For this review, use the dimensioned drawing (mm, ordinates from the lowest corner) and the shaded views. A direction names the side the tool comes from. Coordinates: 2 decimals unless noted, no trailing zeros. Write each loop counter-clockwise with the first axis right and the second up, starting at its lowest first coordinate (ties: lowest second). Pieces come first, ordered by that corner, then holes.
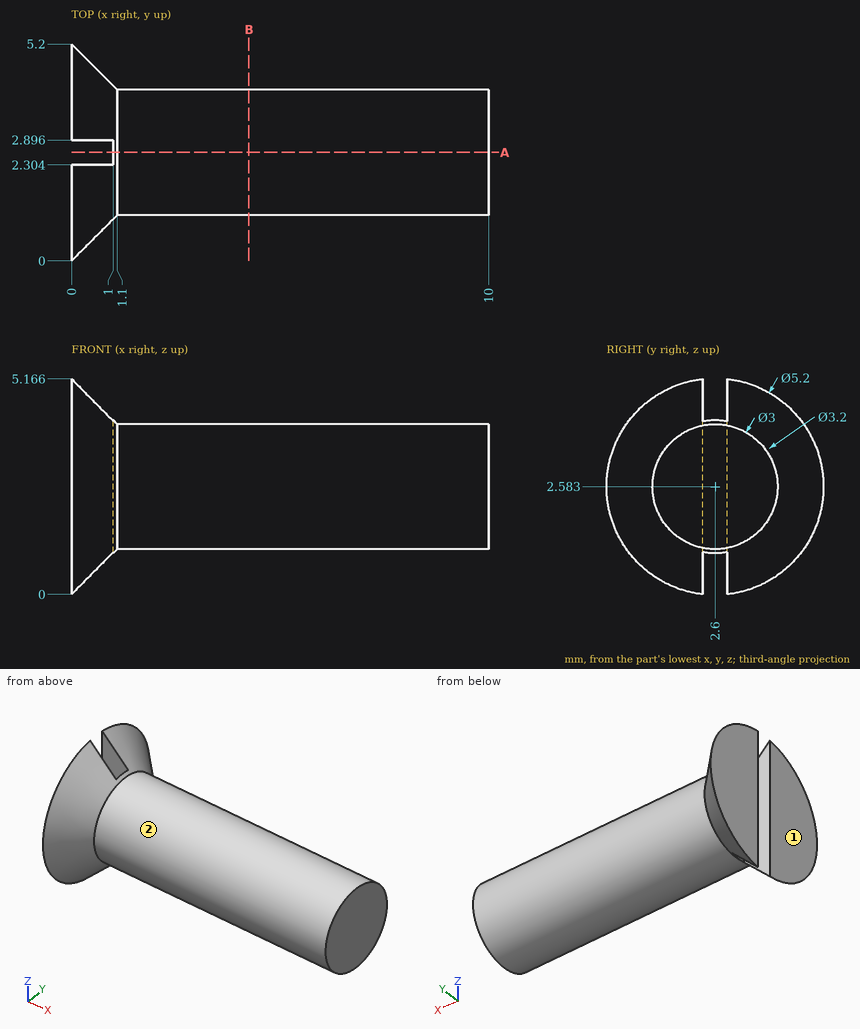
Item 1: Take a section at B-B, the plane x = 4.25. Write out the cut boundary in (y, z).
Solved:
outline: circle Ø3 at (2.6, 2.58)
Item 2: For pin 1 (3 mm diameter, centred on x = 5, z = 1, fed in from +Y); pin 2 (1 mm diameter, centred on x = 7, z = 3.5, fed in from +Y), all flat-tipped, find the tip position at first contact; note any pin that passes through.
Solved:
pin 1: stops at y = 4.1
pin 2: stops at y = 4.04
Item 3: To check wall thickness, follow line 1 along Z through (x, y) = (8.5, 2.7); line 2 along Z through (x, y) = (1.75, 1.7); line 3 along Y through (x, z) = (8.5, 2.1). State the ranges of each line that lie inside material, in increasing order.
Solved:
line 1: z = 1.09 to 4.08
line 2: z = 1.38 to 3.78
line 3: y = 1.18 to 4.02
Item 4: Machinability: for the marked faces 1 and 2, which of the approach directions +Z, -Z, +X, -X, +Y, -Y give a long, thin tool a straight path to every point of the face, cutting with its end or side? Answer none if there is none.
Solved:
face 1: +Z, -Z, -X, +Y, -Y
face 2: +X
Item 5: Take a section at A-A, the plane y = 2.6. Write out the cut boundary in (x, z).
Solved:
outline: (1, 0.98) - (1.1, 1.08) - (10, 1.08) - (10, 4.08) - (1.1, 4.08) - (1, 4.18) - close
